The model under review builds one solid part; all positions refer to its coordinate system, in mm. Face numbers are marked on the shaded views. A direction names the side the tool comes from. Round coordinates to 2 decimals unless told otherwise and drop trailing zeros. Write each loop counter-clockwise with the first axis right and the second up, starting at its lowest first coordinate (ties: lowest second). Pieces come first, ordered by that corner, then holes. Notation, with made-up numbers: (1, -30) -> (39, -30) arc R34 ccw to (39, 1) -> close; hole circle Ø4 at (-5.75, -12). An arc over 180 degrees is marked (long way). Answer as a JSON object with one key per item and string values. Group by question number.
1) Machinability: for the marked faces 1 and 2, which of the approach directions +Z, -Z, +X, -X, +Y, -Y give a long, thin tool a straight path to every point of the face, cutting with its end or side? Answer none if there is none.
2) To check wall thickness, follow probe 1 along X at (y, z) = (-6, 0); probe 2 along X at (y, z) = (0, 3.75); probe 3 along Y at (x, z) = (-11, 3). State the ranges of each line that lie inside material, in increasing order. Write a range as [from, to].
3) We need section B-B, the plane x = 2.5. Write out the cut boundary in (y, z) (3 decimals), then the cut area to 3 significant figures.
4) We need section A-A, the plane x = -11.25. Write out the cut boundary in (y, z), then the cut area to 3 significant figures.
5) Insertion check: pin 1 Ø4 at (x, y) = (3.5, 1) entering from +Z (3 decimals); pin 2 Ø3 at (x, z) = (-6.5, 1) entering from +Y (3 decimals); pin 3 Ø1.5 at (x, z) = (-11.5, -4) entering from -Y; pin 4 Ø6 at (x, y) = (-8.5, -2.5) entering from +Z. Each pin has a flat end and moves straight along its axis. Give the tip position at first contact, or say it passes through.
from build123d import *

# Parameters (mm, degrees)
SKETCH5_R           = 3.175
BOSS_EXTRUDE3_DEPTH = 25.4
CHAMFER1_SIZE       = 0.77724
BOSS_EXTRUDE4_DEPTH = 3.96875
SKETCH8_OUTSIDE_W   = 129.26
SKETCH8_OUTSIDE_H   = 130.98
SKETCH8_OUTSIDE_R   = 5.55625
CUT_EXTRUDE3_DEPTH  = 31.570540439
CUT_EXTRUDE3_DRAFT  = -60
CUT_EXTRUDE4_DEPTH  = 0.254
CIRPATTERN1_COUNT   = 3


with BuildPart() as part:
    # Sketch5 → Boss-Extrude3 (new body)
    with BuildSketch(Plane(origin=(14.684375, 0, 0), x_dir=(0, 0, -1), z_dir=(1, 0, 0))):
        Circle(SKETCH5_R)
    extrude(amount=-BOSS_EXTRUDE3_DEPTH)

    # Chamfer1
    chamfer1_edges = [part.edges().sort_by_distance(p)[0] for p in [
        (14.684375, 0, 3.175),
    ]]
    chamfer(chamfer1_edges, length=CHAMFER1_SIZE)

    # Sketch6 → Boss-Extrude4 (add)
    with BuildSketch(Plane.ZY.offset(10.715625)):
        Polygon((5.55625, 3.207902433), (0, 6.415804866), (-5.55625, 3.207902433), (-5.55625, -3.207902433), (0, -6.415804866), (5.55625, -3.207902433), align=None)
    extrude(amount=BOSS_EXTRUDE4_DEPTH)


with BuildPart() as cut_extrude3_tool:
    # Sketch8 outside → Cut-Extrude3 (with draft: the straight prism first)
    with BuildSketch(Plane.ZY.offset(14.684375)):
        Rectangle(SKETCH8_OUTSIDE_W, SKETCH8_OUTSIDE_H)
        Circle(SKETCH8_OUTSIDE_R, mode=Mode.SUBTRACT)
    extrude(amount=-CUT_EXTRUDE3_DEPTH)
    # Cut-Extrude3: the draft: its side faces are tilted about the plane it starts from
    cut_extrude3_sides = [cut_extrude3_tool.faces().sort_by_distance(p)[0] for p in [
        (1.100895219, -65.49, 0),
        (1.100895219, 0, 64.63),
        (1.100895219, 65.49, 0),
        (1.100895219, 0, -64.63),
        (1.100895219, 0, -5.55625),
    ]]
    draft(cut_extrude3_sides, Plane.ZY.offset(14.684375), CUT_EXTRUDE3_DRAFT)


with BuildPart() as part_1:
    add(part.part)

    # Cut-Extrude3: cut by cut_extrude3_tool
    add(cut_extrude3_tool.part, mode=Mode.SUBTRACT)

    # Sketch12 → Cut-Extrude4 (cut)
    with BuildSketch(Plane.ZY.offset(14.684375)):
        with BuildLine():
            Line((0.1666875, 4.2783125), (0.1666875, 2.3891875))
            ThreePointArc((0.1666875, 2.3891875), (0, 2.2225), (-0.1666875, 2.3891875))
            Line((-0.1666875, 2.3891875), (-0.1666875, 4.2783125))
            ThreePointArc((-0.1666875, 4.2783125), (0, 4.445), (0.1666875, 4.2783125))
        make_face()
    cut_extrude4 = extrude(amount=-CUT_EXTRUDE4_DEPTH, mode=Mode.SUBTRACT)

    # CirPattern1: Cut-Extrude4 ×3 about axis
    cirpattern1_axis = Axis((0, 0, 0), (1, 0, 0))
    for i in range(1, CIRPATTERN1_COUNT):
        add(cut_extrude4.rotate(cirpattern1_axis, i * 360 / CIRPATTERN1_COUNT), mode=Mode.SUBTRACT)


solid = part_1.part
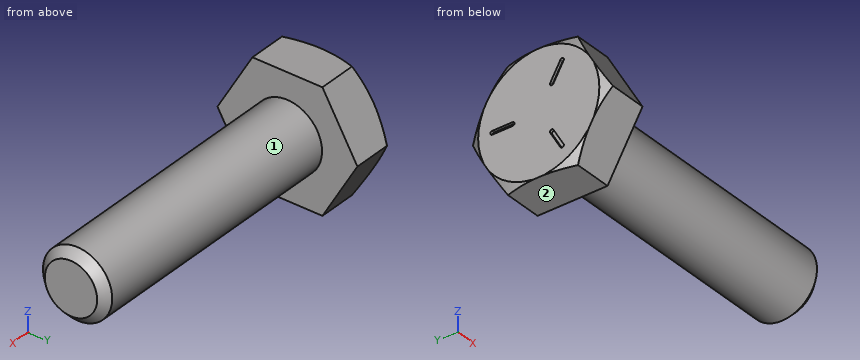
Here are the results:
{
 "1": {"face 1": "+X", "face 2": "-Z, +X, -X, +Y, -Y"},
 "2": {"probe 1": "x = [-14.43, -10.72]", "probe 2": "x = [-14.68, -10.72]", "probe 3": "y = [-4.68, 4.68]"},
 "3": {"outline": "circle Ø6.35 at (0, 0)", "area": "31.7 mm^2"},
 "4": {"outline": "(-6.42, 0) -> (-3.21, -5.56) -> (3.21, -5.56) -> (6.42, 0) -> (3.21, 5.56) -> (-3.21, 5.56) -> close", "area": "107 mm^2"},
 "5": {"pin 1": "stops at z = 3.175", "pin 2": "stops at y = 3.175", "pin 3": "stops at y = -4.54", "pin 4": "stops at z = 5.56"}
}
